Here's how the part is built. I have some questions about the finished solid (model axes, mm). Face numbers are marked on the shaded views. A direction names the side the tool comes from. Give positions to 0.01 mm unless a question says otherwise; leave off trailing zeros. Loops run counter-clockwise (first coordinate to the right, second up) from the corner with the lowest first, then second, coordinate; pieces in that order, holes last. Notation, with made-up numbers: (42.5, -15) - (81.5, -15) arc R10 cw to (81.5, -8) - close; hole circle Ø5 at (60, -7). An arc over 180 degrees is marked (long way). Put each result on its own line as item: value. Start each with the question number.
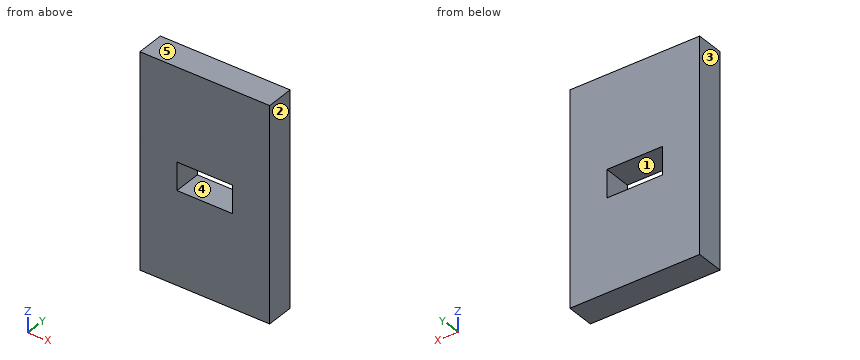
Autodesk Inventor part; units mm, degrees
ref_plane "YZ Plane" through (0, 0, 0) normal (1, 0, 0) x (0, 1, 0)
ref_plane "XZ Plane" through (0, 0, 0) normal (0, 1, 0) x (-1, 0, 0)
ref_plane "XY Plane" through (0, 0, 0) normal (0, 0, 1) x (1, 0, 0)
sketch "Sketch1" plane through (0, 0, 0) normal (0, 0, 1) x (1, 0, 0)
  point P0 (0, 0)
sketch "Sketch2" plane through (0, 0, 0) normal (0, 1, 0) x (-1, 0, 0)
  line L0 (0, 0) -> (-14, 0)
  line L1 (-14, 0) -> (-14, -23)
  line L2 (-14, -23) -> (0, -23)
  line L3 (0, -23) -> (0, 0)
  line L4 (-4, -13) -> (-10, -13)
  line L5 (-10, -13) -> (-10, -10)
  line L6 (-10, -10) -> (-4, -10)
  line L7 (-4, -10) -> (-4, -13)
  dimension "d0" = 14
  dimension "d1" = 23
  dimension "d2" = 6
  dimension "d3" = 3
  dimension "d4" = 10
  dimension "d5" = 4
extrude "Extrusion1" add sketch "Sketch2" along normal blind 3
properties part number "OpenROV 2_2 Horizontal Ducting Brace"
1) Suppose I cut it at B-B on y = 0.3. Please give me the cut outline in (x, z), plus the area to 3 significant figures.
2) Which directions (+Z, -Z, +X, -X, +Y, -Y) give clear straight access to the entire face, cutting with the end or side of a thin tool? Please do the marked faces 1 and 2.
3) Thinking about a two-plate mould opening in Z: for the marked faces 3, 4 and 5, which applies, pulls with the +Z half, pulls with the -Z half, needs draft (parallel to the pull), parting line crosses it, or undercut?
4) I'm going to push a flat-ended pin straight in: P1, Ø3, axis at x = 10.5, z = -14, coming from the -Y side. Where does the tip first touch, or does it pass through?
5) Suppose I cut it at A-A on x = 9.5. Please give me the cut outline in (y, z).
6) I need wall thicknesses on line 1 (X direction, y = 0.45, z = -10.75); line 2 (Z direction, x = 5.75, y = 1.5). Which ranges of each line are inside material? Lowest first, please.
7) Suppose I cut it at C-C on z = -12.75. Please give me the cut outline in (x, y), plus the area to 3 significant figures.
Ans:
1. outline: (0, -23) - (14, -23) - (14, 0) - (0, 0) - close; hole (4, -13) - (10, -13) - (10, -10) - (4, -10) - close
1. area: 304 mm²
2. face 1: +Y, -Y
2. face 2: +Z, -Z, +X, +Y, -Y
3. face 3: needs draft
3. face 4: undercut
3. face 5: pulls with the +Z half
4. P1: stops at y = 0
5. outline: (0, -23) - (3, -23) - (3, -13) - (0, -13) - close; (0, -10) - (3, -10) - (3, 0) - (0, 0) - close
6. line 1: x = 0 to 4, 10 to 14
6. line 2: z = -23 to -13, -10 to 0
7. outline: (0, 0) - (4, 0) - (4, 3) - (0, 3) - close; (10, 0) - (14, 0) - (14, 3) - (10, 3) - close
7. area: 24.0 mm²
